Source: CAD feature listing. Evaluate the final solid. Frame: model axes, mm. A direction names the side the tool comes from. Round coordinates to 2 decimals unless told otherwise and drop trailing zeros. Write each loop counter-clockwise with the first axis right and the second up, starting at its lowest first coordinate (ties: lowest second). Pieces come first, ordered by that corner, then holes. Notation, with made-up numbers: (32.25, 30.5) - (36.25, 30.5) arc R11 ccw to (36.25, 48.5) - close; hole circle Ø3 at (67.5, -5). An arc over 180 degrees is marked (long way). Write item = value, one per line. Start each with the question number.
```python
from build123d import *

# Parameters (mm, degrees)
CORTAR_EXTRUIR1_DEPTH      = 41.890096601
CORTAR_EXTRUIR1_DEPTH_BACK = 41.890096601
CROQUIS2_R                 = 0.5
CORTAR_EXTRUIR2_DEPTH      = 27.400757565
CORTAR_EXTRUIR2_DEPTH_BACK = 27.400757565
CROQUIS3_R                 = 1


with BuildPart() as part:
    # Croquis1 → Revolución1 (revolve)
    with BuildSketch(Plane.XY, mode=Mode.PRIVATE) as revoluci_n1_sk:
        Polygon((0.9, 20), (0.9, 5), (6, 5), (6, 2), (4, 2), (4, -2), (6, -2), (6, -5), (0.9, -5), (0.9, -20), (0, -20), (0, 20), align=None)
    revolve(revoluci_n1_sk.sketch.rotate(Axis((0, 0, 0), (0, 1, 0)), 90), axis=Axis((0, 0, 0), (0, 1, 0)))

    # Croquis2 → Cortar-Extruir1 (cut, two sides: drawn at the far end of the back side and taken through both)
    with BuildSketch(Plane(origin=(0, 20, 0), x_dir=(1, 0, 0), z_dir=(0, 1, 0)).offset(-CORTAR_EXTRUIR1_DEPTH_BACK)):
        with Locations(Location((0, 0, 0), (0, 0, 270))):
            Circle(CROQUIS2_R)
    extrude(amount=CORTAR_EXTRUIR1_DEPTH + CORTAR_EXTRUIR1_DEPTH_BACK, mode=Mode.SUBTRACT)

    # Croquis3 → Cortar-Extruir2 (cut, two sides: drawn at the far end of the back side and taken through both)
    with BuildSketch(Plane(origin=(0, 5, 0), x_dir=(1, 0, 0), z_dir=(0, 1, 0)).offset(-CORTAR_EXTRUIR2_DEPTH_BACK)):
        with Locations(Location((0, 0, 0), (0, 0, 270))):
            Circle(CROQUIS3_R)
    extrude(amount=CORTAR_EXTRUIR2_DEPTH + CORTAR_EXTRUIR2_DEPTH_BACK, mode=Mode.SUBTRACT)


solid = part.part
```
(1) Section A-A (z = 0). Return the cut outline in (x, y).
(2) Section B-B (x = 0). Return the cut outline in (y, z).
(3) Section C-C (y = -1.75). Return the cut outline in (x, z).
(4) Pull-direction query (Y, two-part tool) for faces 3 (the flat face through (3.92, -2, -1.42)), 4 (the flat face through (-0.1, 5, 1.2)), 5 (the cylindrical face through (-1.802, 3.479, -5.723)); classes: +Y half, -Y half, draft (parallel to the pull), parting line (faces both ways), or undercut.
(5) Reachability of faces 1 (the flat face through (3.92, 2, 1.42)), 2 (the flat face through (-0.1, -5, -1.2)) from +Z, -Z, +X, -X, +Y, -Y: full face, straight path, thin tool, end or side. Return the list, or none.
(6) Contact query for flat-ended pins moving along their axis: P1, Ø3, axis at y = -4, z = -2.5, coming from the -X side; P2, Ø2, axis at y = -2, z = 1.5, coming from the +X side. Output: stop coordinate, or through.
(7) Ray query, L1, parallel to X at y = 3, z = 0; L2, parallel to X at y = 0.25, z = 0; L3, parallel to Y at x = -1.5, z = -4.75. Return the intervals inside material, ascending. Write a range as from..to.
(8) Section D-D (x = -4.5). Return the cut outline in (y, z), plus the area to 3 significant figures.
Solution:
q1.outline = (-6, -5) - (-1, -5) - (-1, 5) - (-6, 5) - (-6, 2) - (-4, 2) - (-4, -2) - (-6, -2) - close; (1, -5) - (6, -5) - (6, -2) - (4, -2) - (4, 2) - (6, 2) - (6, 5) - (1, 5) - close
q2.outline = (-5, -6) - (-2, -6) - (-2, -4) - (2, -4) - (2, -6) - (5, -6) - (5, -1) - (-5, -1) - close; (-5, 1) - (5, 1) - (5, 6) - (2, 6) - (2, 4) - (-2, 4) - (-2, 6) - (-5, 6) - close
q3.outline = circle Ø8 at (0, 0); hole circle Ø2 at (0, 0)
q4.face_3 = undercut
q4.face_4 = +Y half
q4.face_5 = draft
q5.face_1 = none
q5.face_2 = +Z, -Z, +X, -X, -Y
q6.P1 = -5.92
q6.P2 = 5.98
q7.L1 = -6..-1, 1..6
q7.L2 = -4..-1, 1..4
q7.L3 = -5..-2, 2..5
q8.outline = (-5, -3.97) - (-2, -3.97) - (-2, 3.97) - (-5, 3.97) - close; (2, -3.97) - (5, -3.97) - (5, 3.97) - (2, 3.97) - close
q8.area = 47.6 mm^2
